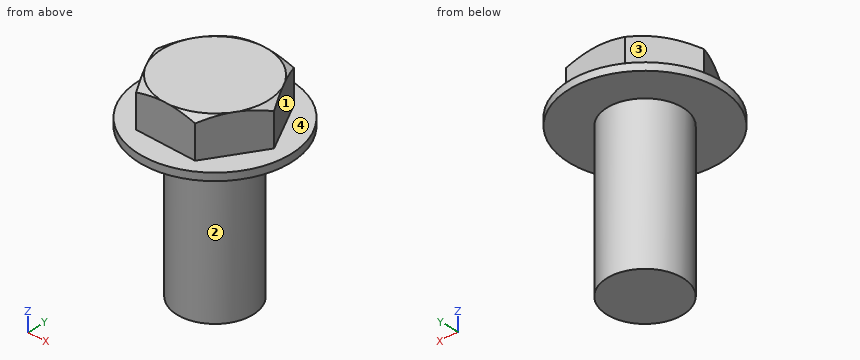
Solid Edge part; units mm, degrees
sketch "Sketch1" plane through (0, 0, 0) normal (0, 0, 1) x (1, 0, 0)
  circle A0 centre (0, 0) radius 5
extrude "Protrusion1" add sketch "Sketch1" against normal blind 0.5
sketch "Sketch2" plane through (0, 0, 0) normal (0, 0, 1) x (1, 0, 0)
  line L0 (-2.0901, -3.459) -> (1.9506, -3.5396)
  line L1 (1.9506, -3.5396) -> (4.0406, -0.0806)
  line L2 (4.0406, -0.0806) -> (2.0901, 3.459)
  line L3 (2.0901, 3.459) -> (-1.9506, 3.5396)
  line L4 (-1.9506, 3.5396) -> (-4.0406, 0.0806)
  line L5 (-4.0406, 0.0806) -> (-2.0901, -3.459)
extrude "ExtrudedProtrusion_2" add sketch "Sketch2" along normal blind 2.5
sketch "Sketch3" plane through (0, 0, -0.5) normal (0, 0, -1) x (1, 0, 0)
  circle A0 centre (0, 0) radius 2.5
extrude "ExtrudedProtrusion_3" add sketch "Sketch3" along normal blind 10
sketch "Sketch4" plane through (-4.0406, 0.0806, 2.5) normal (-0.0199, -0.9998, 0) x (0, 0, -1)
  line L0 (0, 7.5415) -> (0.3126, 8.0829)
  line L1 (0.3126, 8.0829) -> (0, 8.0829)
  line L2 (0, 8.0829) -> (0, 7.5415)
revolve "RevolvedCutout1" cut sketch "Sketch4" angle 360 about axis through (0, 0, 0) along (0, 0, 1)
Model file for the job. Use its own axes, mm. Face numbers are marked on the shaded views. A direction names the side the tool comes from. Give positions to 0.01 mm unless a question says otherwise; leave off trailing zeros. Loops run counter-clockwise (first coordinate to the right, second up) from the corner with the lowest first, then second, coordinate; pieces in that order, holes last. Notation, with made-up numbers: (28, 47.25) - (77, 47.25) arc R21 ccw to (77, 79.25) - close; hole circle Ø5 at (50, 68.5). An arc over 180 degrees is marked (long way). One line per item, written item: value. Start each with the question number.
1. Which spindle directions (+Z, -Z, +X, -X, +Y, -Y) get a long thin tool onto all of the face, cutting with end or side? Do the marked faces 1, 2, 3 and 4. Say none if no direction does.
2. Slice it at C-C (z = -5). List the corners of the cut face in (x, y).
3. Slice it at B-B (y = 4.25). List the corners of the cut face in (x, z), plus the area to 3 significant figures.
4. Probe L1, parallel to Z at x = 4.25, y = 2; L2, parallel to Y at x = 0, z = 1.25; L3, parallel to Y at x = 1.5, z = -6. List the from-to ranges inside material, lowest first. Write a range as from..to.
5. Slice it at A-A (z = -0.25). List the corners of the cut face in (x, y).
6. Pin check, flat tips, straight feed: pin 1 (3 mm diameter, centred on y = 4, z = 0.5, fed in from +X); pin 2 (3 mm diameter, centred on y = -1.5, z = -5.5, fed in from +X); pin 3 (4 mm diameter, centred on y = -1, z = -6.5, fed in from -X). Stop position of each tip, or through.
Solution:
1. face 1: +Z, +X, +Y
1. face 2: -Z
1. face 3: +Z, -X, +Y
1. face 4: +Z
2. outline: circle Ø5 at (0, 0)
3. outline: (-2.63, -0.5) - (2.63, -0.5) - (2.63, 0) - (-2.63, 0) - close
3. area: 2.63 mm^2
4. L1: z = -0.5..0
4. L2: y = -3.5..3.5
4. L3: y = -2..2
5. outline: circle Ø10 at (0, 0)
6. pin 1: stops at x = 4.28
6. pin 2: stops at x = 2.5
6. pin 3: stops at x = -2.5
